```python
from build123d import *

# Parameters (mm, degrees)
SKETCH1_R           = 5.75
SKETCH1_R_2         = 3
BOSS_EXTRUDE1_DEPTH = 12
BOSS_EXTRUDE2_DEPTH = 6
SKETCH3_R           = 1.5
CUT_EXTRUDE1_DEPTH  = 21.199009877


with BuildPart() as part:
    # Sketch1 → Boss-Extrude1 (new body)
    with BuildSketch(Plane.XY):
        Circle(SKETCH1_R)
        Circle(SKETCH1_R_2, mode=Mode.SUBTRACT)
    extrude(amount=BOSS_EXTRUDE1_DEPTH)

    # Sketch2 → Boss-Extrude2 (add)
    with BuildSketch(Plane.XY.offset(12)):
        Polygon((3.464101615, -6), (6.92820323, 0), (3.464101615, 6), (-3.464101615, 6), (-6.92820323, 0), (-3.464101615, -6), align=None)
    extrude(amount=BOSS_EXTRUDE2_DEPTH)

    # Sketch3 → Cut-Extrude1 (cut, through all)
    with BuildSketch(Plane.XY.offset(18)):
        Circle(SKETCH3_R)
    extrude(amount=-CUT_EXTRUDE1_DEPTH, mode=Mode.SUBTRACT)


solid = part.part
```
Verification items for the finished model (mm, model axes). A direction names the side the tool comes from. Round coordinates to 2 decimals unless told otherwise and drop trailing zeros. Write each loop counter-clockwise with the first axis right and the second up, starting at its lowest first coordinate (ties: lowest second). Pieces come first, ordered by that corner, then holes. Notation, with made-up numbers: (-19, 52) -> (-12, 52) arc R23 ccw to (-12, 63) -> close; hole circle Ø10 at (81.25, 24.25). An arc over 180 degrees is marked (long way). Write each question's results on one line, items separated by ' | '. Start each with the question number.
1. Cross-section at D-D (y = -2.25). Enter the section's corners in (x, z), then the cut area to 3 significant figures.
2. Cross-section at C-C (z = 6.75). Enter the section's corners in (x, y).
3. Draft check along Y on faces 3 (the flat face through (-5.172, 3.042, 14.958)), 4 (the flat face through (5.172, -3.042, 14.958)), 5 (the cylindrical face through (-1.5, 0.07, 15.04)), 6 (the flat face through (1.3, -1.3, 12)). Enter one of: +Y half, -Y half, draft (parallel to the pull), parting line (faces both ways), or undercut.
4. Material ranges on probe 1 along Y at (x, z) = (0, 16.1); probe 2 along Y at (x, z) = (0, 8.5); probe 3 along X at (y, z) = (-1, 8.25), recorded low to high. Write a range as from..to.
5. Cross-section at A-A (x = 0). Enter the section's corners in (y, z), then the cut area to 3 significant figures.
6. Cross-section at B-B (y = -0.5). Enter the section's corners in (x, z), then the cut area to 3 significant figures.
7. Set-up check for faces 1 (the cylindrical face through (-0.75, 5.7, 5.92)), 2 (the flat face through (0, -6, 15)): record each of +Z, -Z, +X, -X, +Y, -Y from which the full face is reachable in a straight line by a thin tool's end or side.
8. Depth check by flat-ended pin: P1, Ø3, axis at y = -4.5, z = 9.5, coming from the -X side; P2, Ø2, axis at y = 3, z = 13, coming from the +X side. Enter the tip coordinate at first touch or a pass-through.
Solutions:
1) outline: (-5.63, 12) -> (-5.29, 12) -> (-5.29, 0) -> (-1.98, 0) -> (-1.98, 12) -> (1.98, 12) -> (1.98, 0) -> (5.29, 0) -> (5.29, 12) -> (5.63, 12) -> (5.63, 18) -> (-5.63, 18) -> close | area: 147 mm2
2) outline: circle Ø11.5 at (0, 0); hole circle Ø6 at (0, 0)
3) face 3: +Y half | face 4: -Y half | face 5: undercut | face 6: undercut
4) probe 1: y = -6..-1.5, 1.5..6 | probe 2: y = -5.75..-3, 3..5.75 | probe 3: x = -5.66..-2.83, 2.83..5.66
5) outline: (-6, 12) -> (-5.75, 12) -> (-5.75, 0) -> (-3, 0) -> (-3, 12) -> (-1.5, 12) -> (-1.5, 18) -> (-6, 18) -> close; (1.5, 12) -> (3, 12) -> (3, 0) -> (5.75, 0) -> (5.75, 12) -> (6, 12) -> (6, 18) -> (1.5, 18) -> close | area: 120 mm2
6) outline: (-6.64, 12) -> (-5.73, 12) -> (-5.73, 0) -> (-2.96, 0) -> (-2.96, 12) -> (-1.41, 12) -> (-1.41, 18) -> (-6.64, 18) -> close; (1.41, 12) -> (2.96, 12) -> (2.96, 0) -> (5.73, 0) -> (5.73, 12) -> (6.64, 12) -> (6.64, 18) -> (1.41, 18) -> close | area: 129 mm2
7) face 1: -Z | face 2: +Z, -Z, +X, -X, -Y
8) P1: stops at x = -4.91 | P2: stops at x = 5.77
